Build history of the part. All positions in model axes, mm. Face numbers are marked on the shaded views. Give positions to 0.01 mm unless a question says otherwise; leave off trailing zeros. Loops run counter-clockwise (first coordinate to the right, second up) from the corner with the lowest first, then second, coordinate; pieces in that order, holes last. Notation, with made-up numbers: (-20, 73.25) -> (15, 73.25) arc R21 cw to (15, 78.25) -> close; hole circle Ø8 at (80.5, -37.75). An arc over 180 degrees is marked (long way). Answer as a JSON object with one key per item and string values. Group by question number.
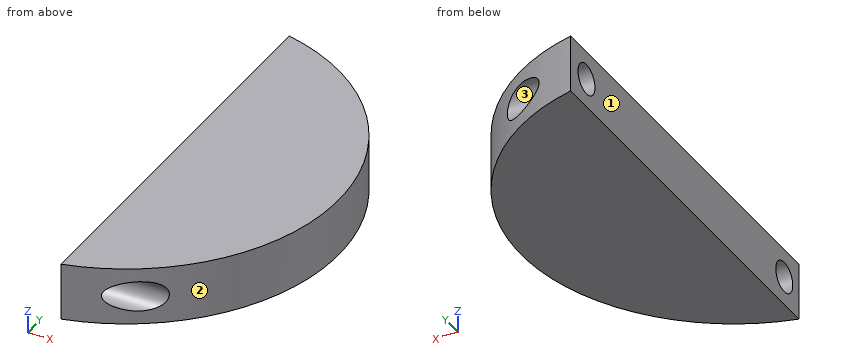
Autodesk Inventor part; units mm, degrees
ref_plane "YZ Plane" through (0, 0, 0) normal (1, 0, 0) x (0, 1, 0)
ref_plane "XZ Plane" through (0, 0, 0) normal (0, 1, 0) x (-1, 0, 0)
ref_plane "XY Plane" through (0, 0, 0) normal (0, 0, 1) x (1, 0, 0)
sketch "Sketch1" plane through (0, 0, 0) normal (0, 0, 1) x (1, 0, 0)
  line L0 (6.2115, -26.7893) -> (6.2115, 26.924)
  line L1 (6.2115, 26.7893) -> (6.2115, -26.7893)
  arc A0 (6.2115, -26.924) -> (6.2115, 26.924) centre (-0.1699, 0) ccw
  line L2 (6.2115, 26.924) -> (6.2115, -26.924)
  point P0 (0, 0)
  point P1 (-5.2115, 24.6247)
extrude "Extrusion1" add sketch "Sketch1" along normal blind 7.5
sketch "Sketch2" plane through (6.2115, -26.924, 0) normal (-1, 0, 0) x (0, 0, 1)
  line L0 (0, 6.9167) -> (7.5, 6.9167)
  line L1 (0, 0) -> (0, 6.9167)
  line L2 (0, 6.9167) -> (7.5, 6.9167)
  line L3 (7.5, 26.7893) -> (7.5, 0)
  line L4 (7.5, 6.9167) -> (7.5, 0)
  line L5 (7.5, 0) -> (0, 0)
  line L6 (7.5, 0) -> (0, 0)
  circle A0 centre (3.75, 3.4583) radius 1
  line L7 (0, 0) -> (0, 53.5786)
  line L8 (0, 53.5786) -> (0, 0)
  line L9 (0, 26.7893) -> (7.5, 26.7893)
  circle A1 centre (3.75, 50.1203) radius 1
  circle A2 centre (3.75, 3.4583) radius 2
  circle A3 centre (3.75, 50.1203) radius 2
  point P0 (0, 26.924)
  point P1 (280.32, 51.414)
  point P2 (4.4851, 4.1363)
  point P3 (4.4851, 2.7804)
  point P4 (3.0149, 4.1363)
  point P5 (3.0149, 2.7804)
  dimension "d2" = 2
  dimension "d5" = 4
  dimension "d6" = 4
extrude "Extrusion2" cut sketch "Sketch2" against normal blind 25.4 contours A0 | A1
extrude "Extrusion3" cut sketch "Sketch2" against normal blind 16.35 contours A2 | A3
scale "Scale1" factors (0.5, 0.5, 0.5) then translate (3.1057, 0, 3.75) bodies 1
properties part number "Contrapeso4"
(1) Probe line 1 along Y through (x, z) = (7.75, 6.25); line 2 along X through (y, z) = (8, 4.7); line 3 along X through (y, z) = (1, 6.7). List the from-to ranges inside material, lowest first. Write a range as [from, to].
(2) Pin check, flat tip, straight feed: pin 1 (2 mm diameter, centred on y = 6.5, z = 6.5, fed in from +X). Stop position of the tip, or through.
(3) Saw through at B-B on y = 11. List the corners of the cut face in (x, z).
(4) Saw through at C-C on x = 7.5. List the corners of the cut face in (y, z) (3 decimals).
(5) Pull direction Y, two halves, no side cores. Call the marked faces 1, 2 and 3: pulls with the +Y half, pulls with the -Y half, needs draft (parallel to the pull), parting line crosses it, or undercut.
(6) Saw through at D-D on x = 11.5. List the corners of the cut face in (y, z) (3 decimals).
(7) Saw through at A-A on z = 6.25. List the corners of the cut face in (x, y), plus the area to 3 significant figures.
Calculated:
{
 "1": {"line 1": "y = [-13, -12.51], [-10.95, 10.82], [12.38, 13]", "line 2": "x = [6.21, 14.31]", "line 3": "x = [6.21, 16.82]"},
 "2": {"pin 1": "stops at x = 15.72"},
 "3": {"outline": "(6.21, 3.75) -> (11.41, 3.75) -> (11.41, 4.82) -> (6.21, 4.82) -> close; (6.21, 6.43) -> (11.41, 6.43) -> (11.41, 7.5) -> (6.21, 7.5) -> close"},
 "4": {"outline": "(-13.09, 3.75) -> (13.09, 3.75) -> (13.09, 7.5) -> (-13.09, 7.5) -> close; hole circle Ø2 at (-11.733, 5.625); hole circle Ø2 at (11.598, 5.625)"},
 "5": {"face 1": "needs draft", "face 2": "parting line crosses it", "face 3": "undercut"},
 "6": {"outline": "(-10.932, 3.75) -> (10.932, 3.75) -> (10.932, 4.879) arc R1 cw to (10.932, 6.371) -> (10.932, 7.5) -> (-10.932, 7.5) -> (-10.932, 6.224) arc R1 cw to (-10.932, 5.026) -> close"},
 "7": {"outline": "(6.21, -13.46) arc R13.83 ccw to (8.92, -12.51) -> (6.21, -12.51) -> close; (6.21, -10.95) -> (11.47, -10.95) arc R13.83 ccw to (11.65, 10.82) -> (6.21, 10.82) -> close; (6.21, 12.38) -> (9.2, 12.38) arc R13.83 ccw to (6.21, 13.46) -> close", "area": "200 mm^2"}
}
